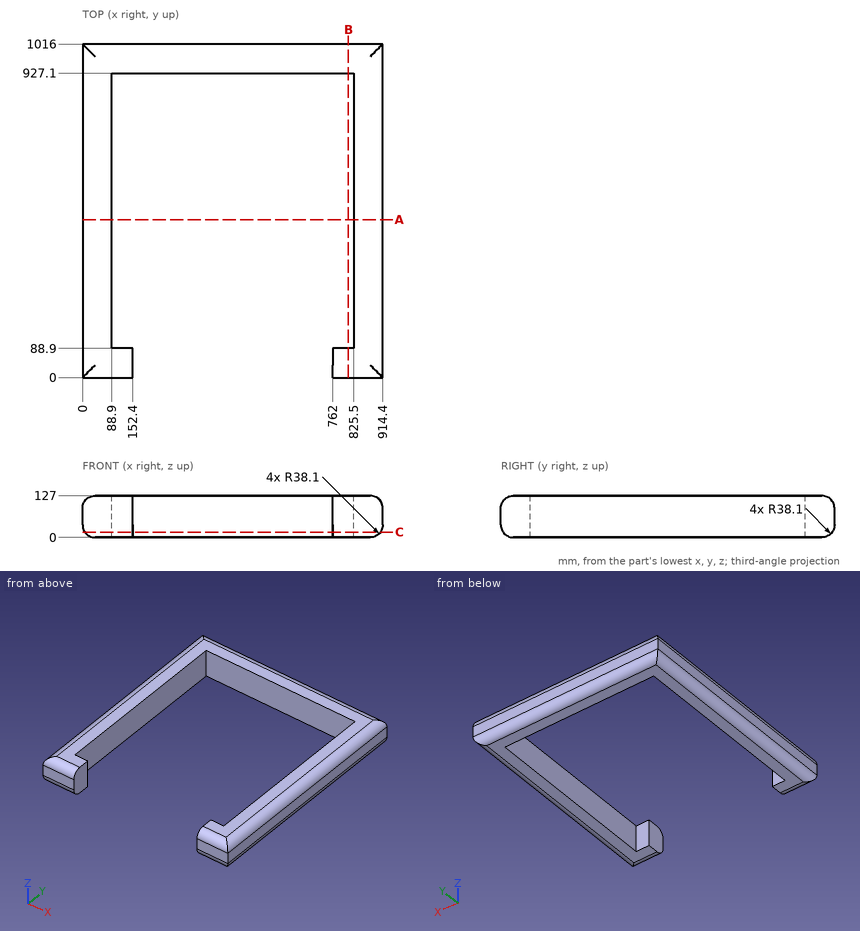
Geometry: see drawing. Coordinates: mm, zero at the bounding-box minimum. Coordinates: 2 decimals unless noted, no trailing zeros. Order: outer loops, then holes, each group sorted by start corner. A loop starts at its lowest first (then second) coordinate and runs counter-clockwise, first axis right, second up. Notation, with made-up numbers: (-17.75, -15.75) - (30.25, -15.75) arc R14 cw to (30.25, -11.75) - close; hole circle Ø1 at (45, 3). An arc over 180 degrees is marked (long way). Return JSON: item names as keys, results as strings.
Q1. First-contact query: pin 1 (5 mm diameter, centred on x = 121, z = 78.5, fed in from -Y); pin 2 (1.5 mm diameter, centred on x = 634, z = 108.5, fed in from +Y). Flat tips, straight axial feed; report the tip coordinate or a pass-through.
The answers:
{"pin 1": "stops at y = 0", "pin 2": "stops at y = 1011.01"}
Q2. Cut plane C-C (z = 16). Return loops of the section in (x, y), then the cut area to 3 significant figures.
The answers:
{"outline": "(7.06, 7.06) - (152.4, 7.06) - (152.4, 88.9) - (88.9, 88.9) - (88.9, 927.1) - (825.5, 927.1) - (825.5, 88.9) - (762, 88.9) - (762, 7.06) - (907.34, 7.06) - (907.34, 1008.94) - (7.06, 1008.94) - close", "area": "235,000 mm2"}
Q3. Cut plane A-A (y = 481). Return loops of the section in (x, z).
The answers:
{"outline": "(0, 38.1) arc R38.1 ccw to (38.1, 0) - (88.9, 0) - (88.9, 127) - (38.1, 127) arc R38.1 ccw to (0, 88.9) - close; (825.5, 0) - (876.3, 0) arc R38.1 ccw to (914.4, 38.1) - (914.4, 88.9) arc R38.1 ccw to (876.3, 127) - (825.5, 127) - close"}
Q4. Cut plane B-B (x = 809.5). Return loops of the section in (y, z).
The answers:
{"outline": "(0, 38.1) arc R38.1 ccw to (38.1, 0) - (88.9, 0) - (88.9, 127) - (38.1, 127) arc R38.1 ccw to (0, 88.9) - close; (927.1, 0) - (977.9, 0) arc R38.1 ccw to (1016, 38.1) - (1016, 88.9) arc R38.1 ccw to (977.9, 127) - (927.1, 127) - close"}
Q5. Ray query, probe 1 along X at (y, z) = (536, 52); probe 2 along Y at (x, z) = (133.5, 65.5); probe 3 along X at (y, z) = (709, 21). Return the intervals inside material, ascending.
The answers:
{"probe 1": "x = 0 to 88.9, 825.5 to 914.4", "probe 2": "y = 0 to 88.9, 927.1 to 1016", "probe 3": "x = 4.05 to 88.9, 825.5 to 910.35"}
